from build123d import *

# Parameters (mm, degrees)
SKETCH1_R           = 4.5
BOSS_EXTRUDE1_DEPTH = 5
CUT_EXTRUDE1_REACH  = 80.329
CUT_EXTRUDE3_REACH  = 59.217
SKETCH6_R           = 1.75
SKETCH8_R           = 15.25
SKETCH8_R_2         = 0.95
CUT_EXTRUDE7_DEPTH  = 0.5


with BuildPart() as part:
    # Sketch1 → Boss-Extrude1 (new body)
    with BuildSketch(Plane(origin=(0, 0, 0), x_dir=(1, 0, 0), z_dir=(0, 1, 0))):
        Polygon((-40.303943114, 15.555205773), (-15.555205773, 40.303943114), (4.694794227, 40.303943114), (24.042773974, 20.955963368), (24.042773974, 0.705963368), (-0.705963368, -24.042773974), (-20.955963368, -24.042773974), (-40.303943114, -4.694794227), align=None)
        with Locations(Location((-11.666118476, -16.618152771, 0), (0, 0, 270))):
            Circle(SKETCH1_R, mode=Mode.SUBTRACT)
        with Locations(Location((16.618152771, 11.666118476, 0), (0, 0, 270))):
            Circle(SKETCH1_R, mode=Mode.SUBTRACT)
        with Locations(Location((-4.595050664, 32.879321912, 0), (0, 0, 270))):
            Circle(SKETCH1_R, mode=Mode.SUBTRACT)
        with Locations(Location((-32.879321912, 4.595050664, 0), (0, 0, 270))):
            Circle(SKETCH1_R, mode=Mode.SUBTRACT)
    extrude(amount=BOSS_EXTRUDE1_DEPTH)

    # Sketch4 → Cut-Extrude1 (cut, up to next)
    with BuildSketch(Plane(origin=(22.499368671, 0, -22.499368671), x_dir=(-0.7071067811865465, 0, -0.7071067811865487), z_dir=(0.7071067811865487, 0, -0.7071067811865465)), mode=Mode.PRIVATE) as cut_extrude1_sk1:
        with BuildLine():
            Line((13.998382969, 5), (8.998382969, 5))
            ThreePointArc((8.998382969, 5), (11.498382969, 2.5), (13.998382969, 5))
        make_face()
    cut_extrude1_tool1 = extrude(cut_extrude1_sk1.sketch, amount=-CUT_EXTRUDE1_REACH, mode=Mode.PRIVATE) & part.part
    add(cut_extrude1_tool1.solids().sort_by_distance((14.368784, 3.938967, -30.629953))[0], mode=Mode.SUBTRACT)

    # Sketch6 → Cut-Extrude3 (cut, up to next)
    with BuildSketch(Plane(origin=(0, 5, 0), x_dir=(1, 0, 0), z_dir=(0, 1, 0)), mode=Mode.PRIVATE) as cut_extrude3_sk1:
        with Locations(Location((-23.686933757, 23.686933757, 0), (0, 0, 270))):
            Circle(SKETCH6_R)
    cut_extrude3_tool1 = extrude(cut_extrude3_sk1.sketch, amount=-CUT_EXTRUDE3_REACH, mode=Mode.PRIVATE) & part.part
    # Sketch6 → Cut-Extrude3 (cut, up to next)
    with BuildSketch(Plane(origin=(0, 5, 0), x_dir=(1, 0, 0), z_dir=(0, 1, 0)), mode=Mode.PRIVATE) as cut_extrude3_sk2:
        with Locations(Location((7.425764616, -7.425764616, 0), (0, 0, 270))):
            Circle(SKETCH6_R)
    cut_extrude3_tool2 = extrude(cut_extrude3_sk2.sketch, amount=-CUT_EXTRUDE3_REACH, mode=Mode.PRIVATE) & part.part
    add(cut_extrude3_tool1.solids().sort_by_distance((-23.686934, 5, -23.686934))[0], mode=Mode.SUBTRACT)
    add(cut_extrude3_tool2.solids().sort_by_distance((7.425765, 5, 7.425765))[0], mode=Mode.SUBTRACT)

    # Sketch8 → Cut-Extrude7 (cut)
    # profile 1 of 3: a face of its own
    with BuildSketch(Plane.XZ):
        with Locations((-8.13058457, -8.13058457)):
            Circle(SKETCH8_R)
    # profile 2 of 3: a face of its own
    with BuildSketch(Plane.XZ):
        with BuildLine():
            Line((-23.156603671, 2.652793843), (-21.615780603, -1.009349568))
            ThreePointArc((-21.615780603, -1.009349568), (-18.913962984, 2.652793843), (-15.251819573, 5.354611462))
            Line((-15.251819573, 5.354611462), (-18.913962984, 6.89543453))
            ThreePointArc((-18.913962984, 6.89543453), (-23.156603671, 6.89543453), (-23.156603671, 2.652793843))
        make_face()
        with Locations(Location((-21.035283327, 4.774114186, 0), (0, 0, 270))):
            Circle(SKETCH8_R_2, mode=Mode.SUBTRACT)
    # profile 3 of 3: a face of its own
    with BuildSketch(Plane.XZ):
        with BuildLine():
            Line((-1.009349568, -21.615780603), (2.652793843, -23.156603671))
            ThreePointArc((2.652793843, -23.156603671), (6.89543453, -23.156603671), (6.89543453, -18.913962984))
            Line((6.89543453, -18.913962984), (5.354611462, -15.251819573))
            ThreePointArc((5.354611462, -15.251819573), (2.652793843, -18.913962984), (-1.009349568, -21.615780603))
        make_face()
        with Locations(Location((4.774114186, -21.035283327, 0), (0, 0, 270))):
            Circle(SKETCH8_R_2, mode=Mode.SUBTRACT)
    extrude(amount=-CUT_EXTRUDE7_DEPTH, mode=Mode.SUBTRACT)


solid = part.part
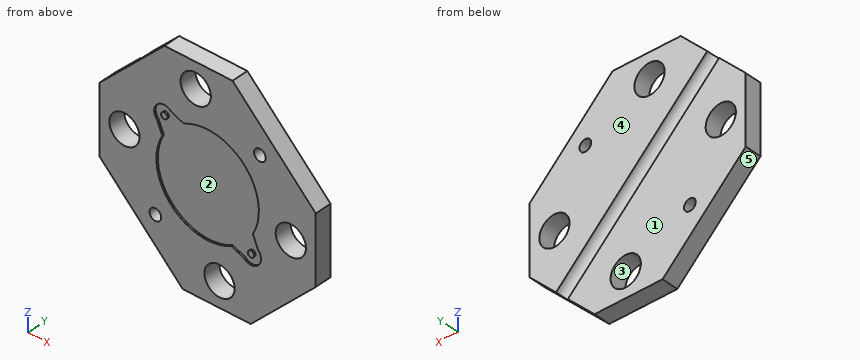
Verification items for the finished model (mm, model axes). Face numbers are marked on the shaded views. A direction names the side the tool comes from. Round coordinates to 2 decimals unless told otherwise and drop trailing zeros. Loops run counter-clockwise (first coordinate to the right, second up) from the corner with the lowest first, then second, coordinate; pieces in that order, holes last. Notation, with made-up numbers: (36, -2) - (93, -2) arc R19 cw to (93, 29) - close; hole circle Ø4 at (-18.5, -14). An arc over 180 degrees is marked (long way). Use a Markdown table: item, result. Add a question column.
1. Section check C-C, the plane x = -34. Record the boundary of the cut face in (y, z).
2. Access from +Z, -Z, +X, -X, +Y, -Y to the whole of each face (thin tool, end or side, straight path). Record for the marked faces 1 and 2.
3. Section check B-B, the plane z = 18.5. Record the boundary of the cut face in (x, y), plus the area to 3 significant figures.
4. Section check A-A, the plane y = 3.85. Record the boundary of the cut face in (x, z).
5. Release check for a two-part mould opening along Z. For the marked faces 3, 4 and 5 record: released by +Z, released by -Z, zero draft, split by the parting line, or undercut.
6. Thickness scan on probe 1 along X at (y, z) = (3.9, -24); probe 2 along X at (y, z) = (3.4, -15.5); probe 3 along Z at (x, y) = (8, 4). Record the ranges inside material, lowest first. Write a range as [from, to].
7. Gauge pin test, flat ends, axial feed: pin 1 (1.5 mm diameter, centred on x = 9.5, y = 4.5, fed in from -Z); pin 2 (4 mm diameter, centred on x = 13, z = -29.5, fed in from +Y). Record the tip position at first contact, or that the pin passes through.
Checks:
| question | item | result |
|---|---|---|
| 1 | outline | (0, -21.86) - (5, -21.86) - (5, -8.95) - (0, -8.95) - close; (0, -0.24) - (5, -0.24) - (5, 11) - (0, 11) - close |
| 2 | face 1 | +Z, -Z, +X, -X, +Y |
| 2 | face 2 | -Y |
| 3 | outline | (-26.5, 0) - (-15.75, 0) - (-15.75, 5) - (-26.5, 5) - close; (-7.58, 0) - (4.84, 0) - (4.84, 5) - (-7.58, 5) - close |
| 3 | area | 116 mm^2 |
| 4 | outline | (-40.3, -15.56) - (-15.56, -40.3) - (4.69, -40.3) - (12.8, -32.2) - (-32.2, 12.8) - (-40.3, 4.69) - close; (-29.06, 15.94) - (15.94, -29.06) - (24.04, -20.96) - (24.04, -0.71) - (-0.71, 24.04) - (-20.96, 24.04) - close; hole circle Ø9 at (-32.88, -4.6); hole circle Ø3.5 at (-23.69, -23.69); hole circle Ø9 at (-11.67, 16.62); hole circle Ø9 at (-4.6, -32.88); hole circle Ø3.5 at (7.43, 7.43); hole circle Ø9 at (16.62, -11.67) |
| 5 | face 3 | undercut |
| 5 | face 4 | zero draft |
| 5 | face 5 | released by -Z |
| 6 | probe 1 | x = [-31.86, -25.41], [-21.97, 4.56], [10.91, 21] |
| 6 | probe 2 | x = [-40.3, -3.48], [1.96, 14.26], [18.97, 24.04] |
| 6 | probe 3 | z = [-37, -27.5], [-21.02, 5.77], [9.08, 15.34] |
| 7 | pin 1 | stops at z = -36.25 |
| 7 | pin 2 | stops at y = 3.76 |
